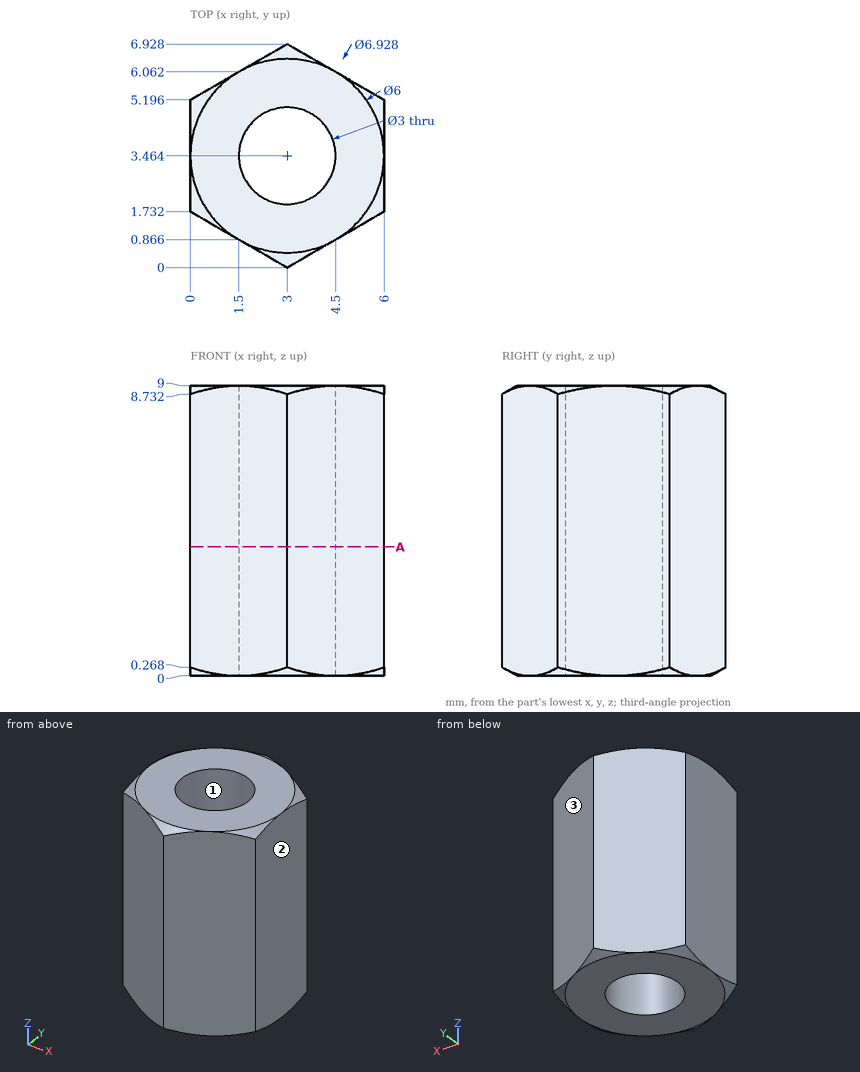
The figure shows three views and two pictorial views of one solid part (mm, origin at its lowest corner). Answer the questions. Round coordinates to 2 decimals unless told otherwise and drop trailing zeros. Order: outer loops, then holes, each group sorted by start corner. A loop starts at its lowest first (then second) coordinate and runs counter-clockwise, first axis right, second up. Notation, with made-up numbers: (39.25, 25.5) -> (93.25, 25.5) arc R20 ccw to (93.25, 59.5) -> close; hole circle Ø2 at (-14.5, -10). An arc over 180 degrees is marked (long way). Put each result on its own line as item: value.
Q1. Section A-A, the plane z = 4 is taken. Write down the section's boundary in (x, y), and give its area (3 significant figures).
Results list:
outline: (0, 1.73) -> (3, 0) -> (6, 1.73) -> (6, 5.2) -> (3, 6.93) -> (0, 5.2) -> close; hole circle Ø3 at (3, 3.46)
area: 24.1 mm^2
Q2. Determine the mould class of the marked faces 1, 2 and 3 for opening direction Y: pulls with the +Y half, pulls with the -Y half, needs draft (parallel to the pull), parting line crosses it, or undercut.
Results list:
face 1: undercut
face 2: needs draft
face 3: pulls with the +Y half
Q3. Consider line 1 along X through (y, z) = (4.5, 8.25) (1 decimal); line 2 along Y through (x, z) = (2.95, 5.75) (1 decimal); line 3 along Y through (x, z) = (5, 7) (1 decimal). Determine where each line is inside the solid, lowest interval first.
Results list:
line 1: 0 to 1.9, 4.1 to 6
line 2: 0 to 2, 5 to 6.9
line 3: 1.2 to 5.8
